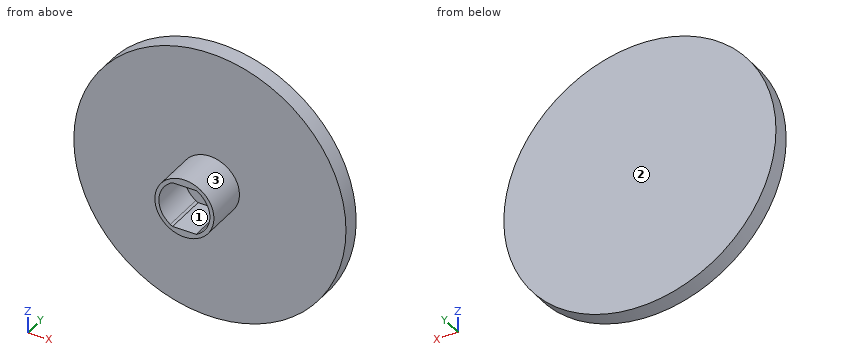
from build123d import *

# Parameters (mm, degrees)
F0_R     = 25.4
F1_DEPTH = 3.175
F2_R     = 5.516158
F3_DEPTH = 7.9375


with BuildPart() as f1:
    # F0 (on Front) → F1 (new body)
    with BuildSketch(Plane.XZ):
        Circle(F0_R)
    extrude(amount=F1_DEPTH)

    # F2 (on face) → F3 (join)
    with BuildSketch(Plane.XZ.offset(3.175)):
        Circle(F2_R)
        with BuildLine():
            ThreePointArc((-2.632571, 3.96875), (-2.420731, 4.101398), (-2.202224, 4.22275))
            Line((-2.202224, 4.22275), (2.202224, 4.22275))
            ThreePointArc((2.202224, 4.22275), (2.420731, 4.101398), (2.632571, 3.96875))
            ThreePointArc((2.632571, 3.96875), (4.7625, 0), (2.632571, -3.96875))
            ThreePointArc((2.632571, -3.96875), (2.420731, -4.101398), (2.202224, -4.22275))
            Line((2.202224, -4.22275), (-2.202224, -4.22275))
            ThreePointArc((-2.202224, -4.22275), (-2.420731, -4.101398), (-2.632571, -3.96875))
            ThreePointArc((-2.632571, -3.96875), (-4.7625, 0), (-2.632571, 3.96875))
        make_face(mode=Mode.SUBTRACT)
    extrude(amount=F3_DEPTH)


solid = f1.part
Work out the finished part from the listing and answer in its coordinate system (mm). Face numbers are marked on the shaded views. Coordinates: 2 decimals unless noted, no trailing zeros. Write each loop counter-clockwise with the first axis right and the second up, starting at its lowest first coordinate (ties: lowest second). Pieces come first, ordered by that corner, then holes. Notation, with made-up numbers: M -16.75,87.25 L 11.25,87.25 A10 ccw 11.25,104.25 Z; hole C 88,-0.5 d8. An arc over 180 degrees is marked long. Write item = value, one per line.
1. The part is cut by section A-A (y = -7.5). Determine the outline of the cut face in (x, z) (1 decimal), then the cut area to 3 significant figures.
Solution:
outline = C 0,0 d11; hole M -2.6,-4 A4.8 ccw -2.2,-4.2 L 2.2,-4.2 A4.8 ccw 2.6,-4 A4.8 ccw 2.6,4 A4.8 ccw 2.2,4.2 L -2.2,4.2 A4.8 ccw -2.6,4 A4.8 ccw Z
area = 27.5 mm2
2. Straight lines are drawn through the part: line 1 (Y direction, x = -5.5, z = -3.5) (3 decimals); line 2 (Z direction, x = 2, y = -9.5); line 3 (X direction, y = -4.5, z = -4). For each, find the intervals that lie inside material, in ascending order. Write a range as from..to.
Solution:
line_1 = -3.175..0
line_2 = -5.14..-4.22, 4.22..5.14
line_3 = -3.8..-2.58, 2.58..3.8
3. The part is cut by section D-D (y = -1.5). Determine the outline of the cut face in (x, z).
Solution:
outline = C 0,0 d50.8
4. The part is cut by section C-C (z = 0). Determine the outline of the cut face in (x, y) (1 decimal), then the cut area to 3 significant figures.
Solution:
outline = M -25.4,-3.2 L -5.5,-3.2 L -5.5,-11.1 L -4.8,-11.1 L -4.8,-3.2 L 4.8,-3.2 L 4.8,-11.1 L 5.5,-11.1 L 5.5,-3.2 L 25.4,-3.2 L 25.4,0 L -25.4,0 Z
area = 173 mm2
5. Determine the mould class of the marked faces 1, 2 and 3 for opening direction X: released by +X, released by -X, zero draft, split by the parting line, or undercut.
Solution:
face_1 = undercut
face_2 = zero draft
face_3 = split by the parting line
6. Flat-ended cylindrical pins translate along their axes: pin 1 (4 mm diameter, centred on y = -3.5, z = -11.5, fed in from -X); pin 2 (3 mm diameter, centred on x = -1, z = -17.5, fed in from +Y); pin 3 (4 mm diameter, centred on x = -14.5, z = 15.5, fed in from -Y) (3 decimals); pin 4 (1.5 mm diameter, centred on y = -1.5, z = 20, fed in from +X). Find the tip coordinate at first contact, or state that the pin passes through.
Solution:
pin_1 = -23.55
pin_2 = 0
pin_3 = -3.175
pin_4 = 16.57
7. The part is cut by section B-B (x = 0). Determine the outline of the cut face in (y, z) (1 decimal).
Solution:
outline = M -11.1,-5.5 L -3.2,-5.5 L -3.2,-25.4 L 0,-25.4 L 0,25.4 L -3.2,25.4 L -3.2,5.5 L -11.1,5.5 L -11.1,4.2 L -3.2,4.2 L -3.2,-4.2 L -11.1,-4.2 Z
